Could you check a few things on this model? Use its own coordinates, in mm. A direction names the side the tool comes from. Give positions to 0.01 mm unless a question says otherwise; leave off trailing zeros. Order: outer loops, then holes, each group sorted by start corner. A loop starts at its lowest first (then second) coordinate and runs counter-clockwise, first axis right, second up. Notation, with made-up numbers: M 7.5,31.5 L 25.5,31.5 A19 ccw 25.5,62.5 Z; hole C 51,83.5 d4. An arc over 180 degrees is marked long. Use a Markdown table: item, result. Add a question column.
```python
from build123d import *

# Parameters (mm, degrees)
ESQUISSE1_R             = 10.45
BASE_EXTRUSION_DEPTH    = 1.5
ESQUISSE2_R             = 10.15
BOSS_EXTRU_1_DEPTH      = 3
ESQUISSE4_R             = 0.9
ENL_V_MAT_EXTRU_2_DEPTH = 16.448462707
BOSS_EXTRU_3_DEPTH      = 2
ESQUISSE3_R             = 1.01
ENL_V_MAT_EXTRU_1_DEPTH = 17.144813409
ESQUISSE7_W             = 2.8
ESQUISSE7_H             = 0.3
BOSS_EXTRU_4_DEPTH      = 5
CONG_1_R                = 1.39
ESQUISSE8_R             = 0.5
ENL_V_MAT_EXTRU_3_DEPTH = 22.489823173
ESQUISSE9_R             = 1.129243381
ESQUISSE9_W             = 2.119235508
ESQUISSE9_H             = 2.258658896
ENL_V_MAT_EXTRU_4_DEPTH = 1


with BuildPart() as part:
    # Esquisse1 → Base-Extrusion (new body)
    with BuildSketch(Plane.XY):
        Circle(ESQUISSE1_R)
    extrude(amount=BASE_EXTRUSION_DEPTH)

    # Esquisse2 → Boss.-Extru.1 (add)
    with BuildSketch(Plane.XY.offset(1.5)):
        Circle(ESQUISSE2_R)
    extrude(amount=BOSS_EXTRU_1_DEPTH)

    # Esquisse4 (on Front Plane) → Enlèv. mat.-Extru.2 (cut, through all)
    with BuildSketch(Plane.XY):
        with Locations((-5.5, 0)):
            Circle(ESQUISSE4_R)
        with Locations(Location((5.5, 0, 0), (0, 0, 180))):
            Circle(ESQUISSE4_R)
    extrude(amount=ENL_V_MAT_EXTRU_2_DEPTH, mode=Mode.SUBTRACT)

    # Esquisse6 → Boss.-Extru.3 (add)
    with BuildSketch(Plane(origin=(0, 0, 0), x_dir=(-1, 0, 0), z_dir=(0, 0, -1))):
        with BuildLine():
            Line((2.327994108, 2.016641622), (2.327994108, -2.016641622))
            ThreePointArc((2.327994108, -2.016641622), (-3.08, 0), (2.327994108, 2.016641622))
        make_face()
    extrude(amount=BOSS_EXTRU_3_DEPTH)

    # Esquisse3 → Enlèv. mat.-Extru.1 (cut, through all)
    with BuildSketch(Plane.XY.offset(4.5)):
        Circle(ESQUISSE3_R)
    extrude(amount=-ENL_V_MAT_EXTRU_1_DEPTH, mode=Mode.SUBTRACT)

    # Esquisse7 → Boss.-Extru.4 (add)
    with BuildSketch(Plane(origin=(0, 0, 0), x_dir=(-1, 0, 0), z_dir=(0, 0, -1))):
        with Locations((0, 7.5)):
            Rectangle(ESQUISSE7_W, ESQUISSE7_H)
        with Locations((0, -7.5)):
            Rectangle(ESQUISSE7_W, ESQUISSE7_H)
    extrude(amount=BOSS_EXTRU_4_DEPTH)

    # Congé1
    cong_1_edges = [part.edges().sort_by_distance(p)[0] for p in [
        (-1.4, -7.5, -5),
        (1.4, -7.5, -5),
        (1.4, 7.5, -5),
        (-1.4, 7.5, -5),
    ]]
    fillet(cong_1_edges, radius=CONG_1_R)

    # Esquisse8 → Enlèv. mat.-Extru.3 (cut, through all)
    with BuildSketch(Plane(origin=(0, 7.65, 0), x_dir=(-1, 0, 0), z_dir=(0, 1, 0))):
        with Locations(Location((0, -3.6, 0), (0, 0, 90))):
            Circle(ESQUISSE8_R)
    extrude(amount=-ENL_V_MAT_EXTRU_3_DEPTH, mode=Mode.SUBTRACT)

    # Esquisse9 → Enlèv. mat.-Extru.4 (cut)
    with BuildSketch(Plane(origin=(0, 0, 0), x_dir=(-1, 0, 0), z_dir=(0, 0, -1))):
        with Locations((3.625008105, 7.082708144)):
            Circle(ESQUISSE9_R)
        with Locations((-3.875970205, -6.789919028)):
            Rectangle(ESQUISSE9_W, ESQUISSE9_H)
    extrude(amount=-ENL_V_MAT_EXTRU_4_DEPTH, mode=Mode.SUBTRACT)


solid = part.part
```
1) Suppose I cut it at B-B on y = 0. Please give me the cut outline in (x, z).
2) We'd pull the mould along Y, two halves only. Please class faces 1 (the face through (0, -7.65, -2)), 2 (the face through (0, 7.65, -2)), 3 (the face through (0, -7.35, -2)): pulls with the +Y half, pulls with the -Y half, needs draft (parallel to the pull), parting line crosses it, or undercut.
3) Please list where these lines run through material, in increasing order: line 1 (Y direction, x = 0, z = 3); line 2 (X direction, y = 0.75, z = 4); line 3 (Y direction, x = 0.5, z = -2.75). Write a range as from..to.
4) Suppose I cut it at C-C on x = 6. Please give me the cut outline in (y, z), and give its area (3 significant figures).
5) For faces 4 (the face through (2.816, -6.8, 0.5)), 5 (the face through (0.963, 0.303, 1.296)), 6 (the face through (-8.05, -6.18, 2.98)), which set-ups out of +Z, -Z, +X, -X, +Y, -Y let a thin tool reach every point of the face, with its end or its side?
6) For pin 1 (0.5 mm diameter, centred on x = 4.5, z = 0.5, fed in from -Y); pin 2 (1.5 mm diameter, centred on x = 7, y = -3, fed in from -Z); pin 3 (0.6 mm diameter, centred on x = 4, y = -7, fed in from -Z); pin 4 (1.6 mm diameter, centred on x = 0, y = 0, fed in from +Z), each with a flat end and sliding along its axis, tell me the tip position at first contact or that it passes through.
7) Suppose I cut it at D-D on z = -2.5. Please give me the cut outline in (x, y).
8) Suppose I cut it at A-A on z = -1. Please give me the cut outline in (x, y).
Values found:
| question | item | result |
|---|---|---|
| 1 | outline | M -10.45,0 L -6.4,0 L -6.4,4.5 L -10.15,4.5 L -10.15,1.5 L -10.45,1.5 Z; M -4.6,0 L -2.33,0 L -2.33,-2 L -1.01,-2 L -1.01,4.5 L -4.6,4.5 Z; M 1.01,-2 L 3.08,-2 L 3.08,0 L 4.6,0 L 4.6,4.5 L 1.01,4.5 Z; M 6.4,0 L 10.45,0 L 10.45,1.5 L 10.15,1.5 L 10.15,4.5 L 6.4,4.5 Z |
| 2 | face 1 | pulls with the -Y half |
| 2 | face 2 | pulls with the +Y half |
| 2 | face 3 | undercut |
| 3 | line 1 | y = -10.15..-1.01, 1.01..10.15 |
| 3 | line 2 | x = -10.12..-6, -5..-0.68, 0.68..5, 6..10.12 |
| 3 | line 3 | y = -7.65..-7.35, 7.35..7.65 |
| 4 | outline | M -8.56,0 L -0.75,0 L -0.75,4.5 L -8.19,4.5 L -8.19,1.5 L -8.56,1.5 Z; M 0.75,0 L 8.56,0 L 8.56,1.5 L 8.19,1.5 L 8.19,4.5 L 0.75,4.5 Z |
| 4 | area | 68.1 mm^2 |
| 5 | face 4 | -Z |
| 5 | face 5 | +Z, -Z |
| 5 | face 6 | +Z |
| 6 | pin 1 | stops at y = -9.55 |
| 6 | pin 2 | stops at z = 0 |
| 6 | pin 3 | stops at z = 1 |
| 6 | pin 4 | passes through |
| 7 | outline | M -1.4,-7.65 L 1.4,-7.65 L 1.4,-7.35 L -1.4,-7.35 Z; M -1.4,7.35 L 1.4,7.35 L 1.4,7.65 L -1.4,7.65 Z |
| 8 | outline | M -2.33,-2.02 A3.08 ccw long -2.33,2.02 Z; M -1.4,-7.65 L 1.4,-7.65 L 1.4,-7.35 L -1.4,-7.35 Z; M -1.4,7.35 L 1.4,7.35 L 1.4,7.65 L -1.4,7.65 Z; hole C 0,0 d2.02 |
